The model under review builds one solid part; all positions refer to its coordinate system, in mm. A direction names the side the tool comes from. Give positions to 0.01 mm unless a question says otherwise; leave off trailing zeros. Loops run counter-clockwise (first coordinate to the right, second up) from the corner with the lowest first, then second, coordinate; pieces in that order, holes last. Notation, with made-up numbers: M 21.25,49 L 70.25,49 A24 ccw 70.25,78 Z; hole C 89,-17.75 d1. An arc over 180 degrees is marked long. Write item = value, one per line. Start each with the question number.
1. For pin 1 (2 mm diameter, centred on x = 10, y = -11.5, fed in from +Z); pin 2 (3 mm diameter, centred on y = -11.5, z = -4.5, fed in from +X); pin 3 (3.5 mm diameter, centred on y = -10, z = -6, fed in from -X), all flat-tipped, find the tip position at first contact; note any pin that passes through.
2. We need section C-C on x = -5. Give the boundary of the cut face in (y, z), then the cut area to 3 significant figures.
3. We need section A-A on z = -11.5. Give the boundary of the cut face in (x, y), then the cut area to 3 significant figures.
4. We need section B-B on y = -7.5. Give the boundary of the cut face in (x, z), then the cut area to 3 significant figures.
5. We need section D-D on y = 1. Give the boundary of the cut face in (x, z).
6. For faces 4 (the face through (-13.55, 23.07, -7.89)), 5 (the face through (10.5, -20, -7.9)), 6 (the face through (0, 10, 5)), 7 (the face through (11, -12, -7)), 8 (the face through (15, -4, 0)), list the 3-axis set-ups (+Z, -Z, +X, -X, +Y, -Y) from which the entire face can be reached by the end or side of a thin tool; tool diameter is ignored.
7. Wall thickness on line 1 along X through (y, z) = (-10, -10.5); line 2 along X through (y, z) = (-11.5, 1.25); line 3 along X through (y, z) = (-21.5, -8.25): over which ranges is each line inside the solid? List them lowest first. Write a range as from..to.
8. Draft analysis for pull direction Y (two halves, no side actions). For faces 1 (the face through (0, 25, 1)), 2 (the face through (-1, -16, -7)), 3 (the face through (8, 15, 5)), state which applies: pulls with the +Y half, pulls with the -Y half, needs draft (parallel to the pull), parting line crosses it, or undercut.
from build123d import *

# Parameters (mm, degrees)
BOSS_EXTRUDE1_DEPTH = 3
BOSS_EXTRUDE2_DEPTH = 16
SKETCH3_W           = 16
SKETCH3_H           = 10
BOSS_EXTRUDE3_DEPTH = 4
CUT_EXTRUDE1_DEPTH  = 17
SKETCH5_W           = 2
SKETCH5_H           = 4
SKETCH5_H_2         = 4.422760465
BOSS_EXTRUDE4_DEPTH = 15


with BuildPart() as part:
    # Sketch1 → Boss-Extrude1 (new body)
    with BuildSketch(Plane.XY):
        with BuildLine():
            Line((-13.5, 25), (13.5, 25))
            ThreePointArc((13.5, 25), (14.914213562, 24.414213562), (15.5, 23))
            Line((15.5, 23), (15.5, -23))
            ThreePointArc((15.5, -23), (14.914213562, -24.414213562), (13.5, -25))
            Line((13.5, -25), (-13.5, -25))
            ThreePointArc((-13.5, -25), (-14.914213562, -24.414213562), (-15.5, -23))
            Line((-15.5, -23), (-15.5, 23))
            ThreePointArc((-15.5, 23), (-14.914213562, 24.414213562), (-13.5, 25))
        make_face()
    extrude(amount=BOSS_EXTRUDE1_DEPTH)

    # Sketch2 → Boss-Extrude2 (add)
    with BuildSketch(Plane(origin=(0, 0, 0), x_dir=(-1, 0, 0), z_dir=(0, 0, -1))):
        with BuildLine():
            Line((-12.5, 23.5), (12.5, 23.5))
            ThreePointArc((12.5, 23.5), (13.560660172, 23.060660172), (14, 22))
            Line((14, 22), (14, -16.5))
            Line((14, -16.5), (7, -23.5))
            Line((7, -23.5), (-7, -23.5))
            Line((-7, -23.5), (-14, -16.5))
            Line((-14, -16.5), (-14, 22))
            ThreePointArc((-14, 22), (-13.560660172, 23.060660172), (-12.5, 23.5))
        make_face()
    extrude(amount=BOSS_EXTRUDE2_DEPTH)

    # Sketch3 → Boss-Extrude3 (add)
    with BuildSketch(Plane.XY.offset(3)):
        with Locations((0, 15)):
            Rectangle(SKETCH3_W, SKETCH3_H)
    extrude(amount=BOSS_EXTRUDE3_DEPTH)

    # Sketch4 → Cut-Extrude1 (cut)
    with BuildSketch(Plane.XY.offset(3)):
        Polygon((-12.5, -17), (-7.5, -22), (7.5, -22), (12.5, -17), (12.5, -6), (-12.5, -6), align=None)
    extrude(amount=-CUT_EXTRUDE1_DEPTH, mode=Mode.SUBTRACT)

    # Sketch5 → Boss-Extrude4 (add)
    with BuildSketch(Plane.XY.offset(-14)):
        with Locations((0, -15.680542245)):
            Rectangle(SKETCH5_W, SKETCH5_H)
        with Locations((-10, -11.680542245)):
            Rectangle(SKETCH5_W, SKETCH5_H)
        with Locations((10, -11.680542244)):
            Rectangle(SKETCH5_W, SKETCH5_H_2)
    extrude(amount=BOSS_EXTRUDE4_DEPTH)


solid = part.part
Final values:
q1.pin_1 = 1
q1.pin_2 = 14
q1.pin_3 = -14
q2.outline = M -25,0 L -23.5,0 L -23.5,-16 L 23.5,-16 L 23.5,0 L 25,0 L 25,3 L 20,3 L 20,7 L 10,7 L 10,3 L -6,3 L -6,-14 L -22,-14 L -22,3 L -25,3 Z
q2.area = 670 mm²
q3.outline = M -14,-16.5 L -7,-23.5 L 7,-23.5 L 14,-16.5 L 14,22 A1.5 ccw 12.5,23.5 L -12.5,23.5 A1.5 ccw -14,22 Z; M -11,-13.68 L -9,-13.68 L -9,-9.68 L -11,-9.68 Z; M -1,-17.68 L 1,-17.68 L 1,-13.68 L -1,-13.68 Z; M 9,-13.89 L 11,-13.89 L 11,-9.47 L 9,-9.47 Z; hole M -12.5,-17 L -7.5,-22 L 7.5,-22 L 12.5,-17 L 12.5,-6 L -12.5,-6 Z
q3.area = 916 mm²
q4.outline = M -15.5,0 L -14,0 L -14,-16 L 14,-16 L 14,0 L 15.5,0 L 15.5,3 L 12.5,3 L 12.5,-14 L -12.5,-14 L -12.5,3 L -15.5,3 Z
q4.area = 116 mm²
q5.outline = M -15.5,0 L -14,0 L -14,-16 L 14,-16 L 14,0 L 15.5,0 L 15.5,3 L -15.5,3 Z
q6.face_4 = -Z, -X, +Y
q6.face_5 = -Z, +X, -Y
q6.face_6 = +Z, +X, -X, -Y
q6.face_7 = +Z
q6.face_8 = -Z
q7.line_1 = -14..-12.5, -11..-9, 9..11, 12.5..14
q7.line_2 = -15.5..-12.5, 12.5..15.5
q7.line_3 = -9..-8, 8..9
q8.face_1 = pulls with the +Y half
q8.face_2 = undercut
q8.face_3 = needs draft
